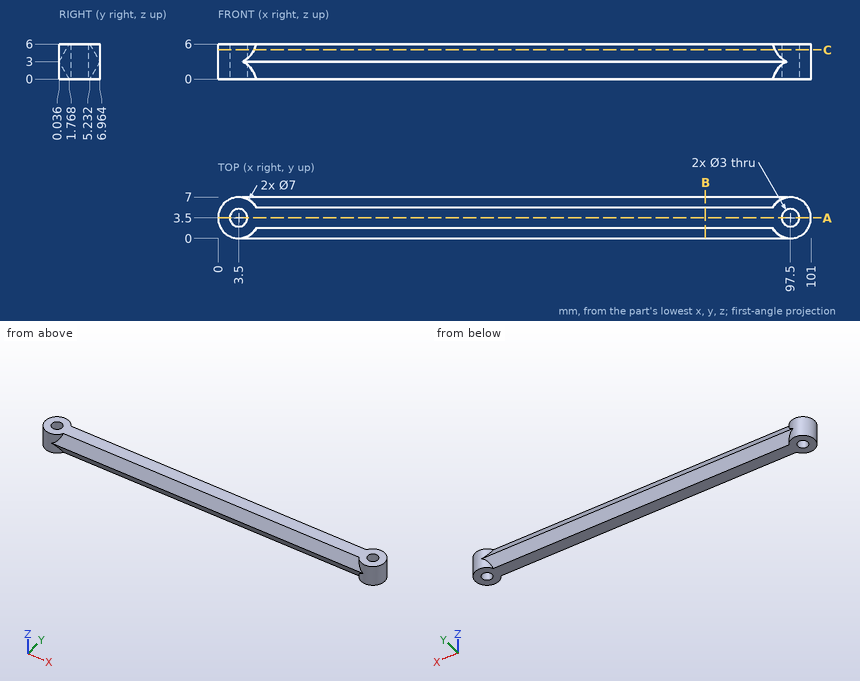
Input: dimensioned drawing with shaded views. Units: mm. Origin: part minimum x, y, z. Give positions to 0.01 mm unless a question says otherwise; leave off trailing zeros. Loops run counter-clockwise (first coordinate to the right, second up) from the corner with the lowest first, then second, coordinate; pieces in that order, holes last. Notation, with made-up numbers: (-38.75, -6.75) -> (-10.75, -6.75) arc R9 ccw to (-10.75, -2.75) -> close; hole circle Ø5 at (-35.5, 89.25). An arc over 180 degrees is marked (long way). Use a Markdown table: item, result. Add a question column.
1) First-contact query: pin 1 (1.5 mm diameter, centred on x = 16, z = 3.5, fed in from -Y); pin 2 (1.8 mm diameter, centred on x = 97.5, y = 3.5, fed in from +Z); pin 3 (4 mm diameter, centred on x = 3.5, y = 3.5, fed in from +Z). Flat tips, straight axial feed; report the tip coordinate or a pass-through.
2) Section query C-C, the plane z = 5. Return the cut outline in (x, y), then the cut area to 3 significant figures.
3) Section query A-A, the plane y = 3.5. Return the cut outline in (x, z).
4) Line query: line 1 along Y through (x, z) = (3.5, 4.45); line 2 along X through (y, z) = (4.25, 4.5); line 3 along X through (y, z) = (4.75, 1.75). Output: solid intervals per line, ascending. Write a range as [from, to].
5) Section query B-B, the plane x = 83. Return the cut outline in (y, z), then the cut area to 3 significant figures.
Numbers:
| question | item | result |
|---|---|---|
| 1 | pin 1 | stops at y = 0.04 |
| 1 | pin 2 | passes through |
| 1 | pin 3 | stops at z = 6 |
| 2 | outline | (6.13, 1.19) -> (94.87, 1.19) arc R3.5 ccw (long way) to (94.87, 5.81) -> (6.13, 5.81) arc R3.5 ccw (long way) to start; hole circle Ø3 at (3.5, 3.5); hole circle Ø3 at (97.5, 3.5) |
| 2 | area | 467 mm2 |
| 3 | outline | (0, 0) -> (2, 0) -> (2, 6) -> (0, 6) -> close; (5, 0) -> (96, 0) -> (96, 6) -> (5, 6) -> close; (99, 0) -> (101, 0) -> (101, 6) -> (99, 6) -> close |
| 4 | line 1 | y = [0, 2], [5, 7] |
| 4 | line 2 | x = [0.08, 2.2], [4.8, 96.2], [98.8, 100.92] |
| 4 | line 3 | x = [0.23, 2.67], [4.33, 96.67], [98.33, 100.77] |
| 5 | outline | (0.04, 3) -> (1.77, 0) -> (5.23, 0) -> (6.96, 3) -> (5.23, 6) -> (1.77, 6) -> close |
| 5 | area | 31.2 mm2 |
